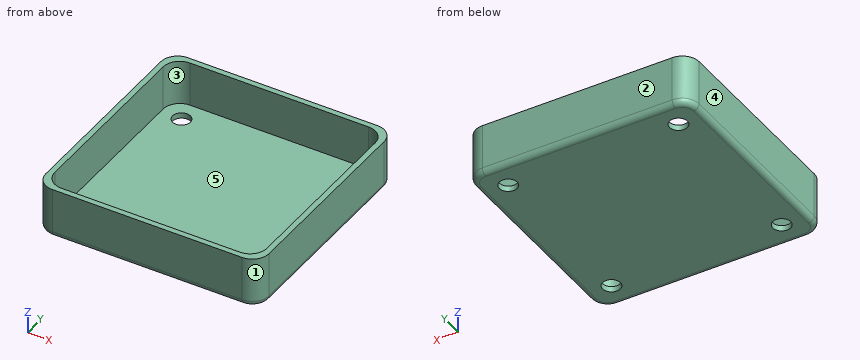
```python
from build123d import *

# Parameters (mm, degrees)
F0_W     = 40
F0_H     = 40
F0_R     = 1.6
F1_DEPTH = 1
F3_DEPTH = 8
F4_R     = 3
F5_R     = 1


with BuildPart() as f1:
    # F0 (on Top) → F1 (new body)
    with BuildSketch(Plane.XY):
        with Locations((-1.320125, -0.328824)):
            Rectangle(F0_W, F0_H)
        with Locations((-16.570125, -15.578824)):
            Circle(F0_R, mode=Mode.SUBTRACT)
        with Locations((13.929875, -15.578824)):
            Circle(F0_R, mode=Mode.SUBTRACT)
        with Locations((-16.570125, 14.921176)):
            Circle(F0_R, mode=Mode.SUBTRACT)
        with Locations((13.929875, 14.921176)):
            Circle(F0_R, mode=Mode.SUBTRACT)
    extrude(amount=F1_DEPTH)

    # F2 (on face) → F3 (join)
    with BuildSketch(Plane.XY.offset(1)):
        Polygon((18.679875, -15.328824), (18.679875, 14.671176), (18.679875, 19.671176), (13.679875, 19.671176), (-16.320125, 19.671176), (-21.320125, 19.671176), (-21.320125, 14.671176), (-21.320125, -15.328824), (-21.320125, -20.328824), (-16.320125, -20.328824), (13.679875, -20.328824), (18.679875, -20.328824), align=None)
        Polygon((17.679875, 18.671176), (17.679875, 14.671176), (17.679875, -15.328824), (17.679875, -19.328824), (13.679875, -19.328824), (-16.320125, -19.328824), (-20.320125, -19.328824), (-20.320125, -15.328824), (-20.320125, 14.671176), (-20.320125, 18.671176), (-16.320125, 18.671176), (13.679875, 18.671176), align=None, mode=Mode.SUBTRACT)
    extrude(amount=F3_DEPTH)

    # F4
    f4_edges = [f1.edges().sort_by_distance(p)[0] for p in [
        (-20.320125, -19.328824, 5),
        (-20.320125, 18.671176, 5),
        (17.679875, 18.671176, 5),
        (17.679875, -19.328824, 5),
        (18.679875, -20.328824, 4.5),
        (18.679875, 19.671176, 4.5),
        (-21.320125, 19.671176, 4.5),
        (-21.320125, -20.328824, 4.5),
    ]]
    fillet(f4_edges, radius=F4_R)

    # F5
    f5_edges = [f1.edges().sort_by_distance(p)[0] for p in [
        (-1.320125, 19.671176, 0),
    ]]
    fillet(f5_edges, radius=F5_R)


solid = f1.part
```
Build history of the part. All positions in model axes, mm. Face numbers are marked on the shaded views. A direction names the side the tool comes from. Give positions to 0.01 mm unless a question says otherwise; leave off trailing zeros. Loops run counter-clockwise (first coordinate to the right, second up) from the corner with the lowest first, then second, coordinate; pieces in that order, holes last. Notation, with made-up numbers: (-32, -3.75) -> (-15, -3.75) arc R25 ccw to (-15, 35.25) -> close; hole circle Ø3 at (87, 66). An arc over 180 degrees is marked (long way). One line per question, with ' | ' between items. Start each with the question number.
1) Cut at A-A (z = 5.25). Give the cut face in (x, y), plus the area to 3 significant figures.
2) Pin check, flat tips, straight feed: pin 1 (2.5 mm diameter, centred on x = 13.93, y = -15.58, fed in from -Z); pin 2 (19 mm diameter, centred on x = 5, y = -1.5, fed in from +Z). Stop position of each tip, or through.
3) Cut at D-D (y = 14). Give the cut face in (x, z), plus the area to 3 significant figures.
4) 3-axis set-ups, long thin cutter, end or side, ignore diameter. For the marked faces 4 and 5: which of +Z, -Z, +X, -X, +Y, -Y reach the whole face in a straight line?
5) Cut at B-B (y = 7). Give the cut face in (x, z).
6) Cut at C-C (x = 9.5). Give the cut face in (y, z).
7) Two-plate mould, pull along Y, no slides. Class the marked faces 1, 2 and 3: released by +Y, released by -Y, zero draft, split by the parting line, or undercut.
8) Probe L1, parallel to Y at x = -17, z = 7.25; L2, parallel to X at y = -2, z = 2.25; L3, parallel to Y at x = 16, z = 4.25. List the from-to ranges inside material, lowest first.
Return value:
1) outline: (-21.32, -17.33) arc R3 ccw to (-18.32, -20.33) -> (15.68, -20.33) arc R3 ccw to (18.68, -17.33) -> (18.68, 16.67) arc R3 ccw to (15.68, 19.67) -> (-18.32, 19.67) arc R3 ccw to (-21.32, 16.67) -> close; hole (-20.32, -16.33) arc R3 ccw to (-17.32, -19.33) -> (14.68, -19.33) arc R3 ccw to (17.68, -16.33) -> (17.68, 15.67) arc R3 ccw to (14.68, 18.67) -> (-17.32, 18.67) arc R3 ccw to (-20.32, 15.67) -> close | area: 156 mm^2
2) pin 1: through | pin 2: z = 1
3) outline: (-21.32, 1) arc R1 ccw to (-20.32, 0) -> (-17.88, 0) -> (-17.88, 1) -> (-20.32, 1) -> (-20.32, 9) -> (-21.32, 9) -> close; (-15.26, 0) -> (12.62, 0) -> (12.62, 1) -> (-15.26, 1) -> close; (15.24, 0) -> (17.68, 0) arc R1 ccw to (18.68, 1) -> (18.68, 9) -> (17.68, 9) -> (17.68, 1) -> (15.24, 1) -> close | area: 50.3 mm^2
4) face 4: +Z, -Z, -X, +Y, -Y | face 5: +Z
5) outline: (-21.32, 1) arc R1 ccw to (-20.32, 0) -> (17.68, 0) arc R1 ccw to (18.68, 1) -> (18.68, 9) -> (17.68, 9) -> (17.68, 1) -> (-20.32, 1) -> (-20.32, 9) -> (-21.32, 9) -> close
6) outline: (-20.33, 1) arc R1 ccw to (-19.33, 0) -> (18.67, 0) arc R1 ccw to (19.67, 1) -> (19.67, 9) -> (18.67, 9) -> (18.67, 1) -> (-19.33, 1) -> (-19.33, 9) -> (-20.33, 9) -> close
7) face 1: released by -Y | face 2: released by +Y | face 3: undercut
8) L1: -20.33 to -19.33, 18.67 to 19.67 | L2: -21.32 to -20.32, 17.68 to 18.68 | L3: -20.31 to -19.02, 18.37 to 19.65
